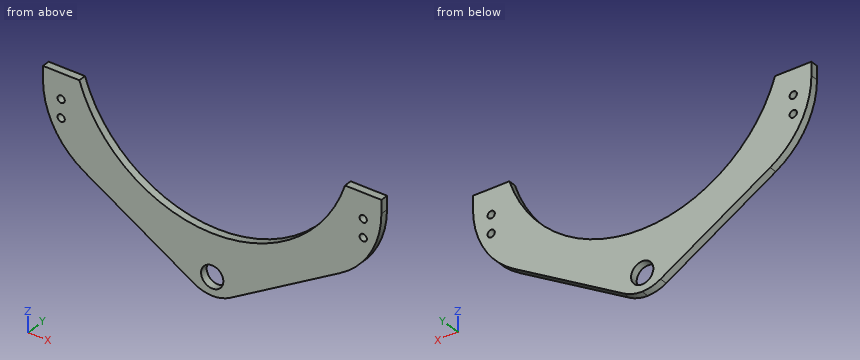
from build123d import *

# Parameters (mm, degrees)
SKETCH1_R           = 4.6
SKETCH1_R_2         = 1.5
BOSS_EXTRUDE2_DEPTH = 3.175


with BuildPart() as part:
    # Sketch1 → Boss-Extrude2 (new body)
    with BuildSketch(Plane(origin=(0, 0, 0), x_dir=(1, 0, 0), z_dir=(0, 1, 0))):
        with BuildLine():
            Line((109.700000056, 0), (117.200000056, 0))
            Line((117.200000056, 0), (124.700000056, 0))
            Line((124.700000056, 0), (124.700000056, 5.554920326))
            ThreePointArc((124.700000056, 5.554920326), (120.146392707, 22.818094267), (107.670447225, 35.589284453))
            Line((107.670447225, 35.589284453), (62.40678526, 62.67187034))
            ThreePointArc((62.40678526, 62.67187034), (58.77003956, 64.238725538), (54.850000028, 64.799300745))
            ThreePointArc((54.850000028, 64.799300745), (50.929960496, 64.238725538), (47.293214796, 62.67187034))
            Line((47.293214796, 62.67187034), (2.029552831, 35.589284453))
            ThreePointArc((2.029552831, 35.589284453), (-10.446392651, 22.818094267), (-15, 5.554920326))
            Line((-15, 5.554920326), (-15, 0))
            Line((-15, 0), (-7.5, 0))
            Line((-7.5, 0), (0, 0))
            ThreePointArc((0, 0), (54.850000028, 39.949878845), (109.700000056, 0))
        make_face()
        with Locations(Location((54.850000028, 57.3, 0), (0, 0, 270))):
            Circle(SKETCH1_R, mode=Mode.SUBTRACT)
        with BuildLine():
            ThreePointArc((117.200000056, 8.9), (115.700000056, 10.4), (117.200000056, 11.9))
            ThreePointArc((117.200000056, 11.9), (118.700000056, 10.4), (117.200000056, 8.9))
        make_face(mode=Mode.SUBTRACT)
        with Locations(Location((117.200000056, 17.9, 0), (0, 0, 270))):
            Circle(SKETCH1_R_2, mode=Mode.SUBTRACT)
        with BuildLine():
            ThreePointArc((-7.5, 8.9), (-9, 10.4), (-7.5, 11.9))
            ThreePointArc((-7.5, 11.9), (-6, 10.4), (-7.5, 8.9))
        make_face(mode=Mode.SUBTRACT)
        with Locations(Location((-7.5, 17.9, 0), (0, 0, 270))):
            Circle(SKETCH1_R_2, mode=Mode.SUBTRACT)
    extrude(amount=BOSS_EXTRUDE2_DEPTH)


solid = part.part
Verification items for the finished model (mm, model axes). Give positions to 0.01 mm unless a question says otherwise; leave off trailing zeros. Write each loop counter-clockwise with the first axis right and the second up, starting at its lowest first coordinate (ties: lowest second). Pieces come first, ordered by that corner, then holes.
(1) Cross-section at A-A (z = -23.5). Enter the section's corners in (x, y) (3 decimals).
(2) Material ranges on line 1 (X direction, y = 1.4, z = -10.4); line 2 (X direction, y = 0.7, z = -17.9); line 3 (X direction, y = 0.85, z = -12), recorded low to high.
(3) Gauge pin test, flat end, axial feed: pin 1 (12 mm diameter, centred on x = 54.85, z = -57.3, fed in from +Y) (3 decimals). Record the tip position at first contact, or that the pin passes through.
(4) Cross-section at C-C (z = -10.4). Enter the section's corners in (x, y) (3 decimals).
(5) Cross-section at D-D (z = -54). Enter the section's corners in (x, y) (3 decimals).
(6) Cross-section at B-B (y = 1.25). Enter the section's corners in (x, z).
Worked out:
1. outline: (-10.05, 0) - (14.534, 0) - (14.534, 3.175) - (-10.05, 3.175) - close; (95.166, 0) - (119.75, 0) - (119.75, 3.175) - (95.166, 3.175) - close
2. line 1: x = -14.66 to -9, -6 to 4.52, 105.18 to 115.7, 118.7 to 124.36
2. line 2: x = -12.75 to -9, -6 to 9.52, 100.18 to 115.7, 118.7 to 122.45
2. line 3: x = -14.4 to 5.45, 104.25 to 124.1
3. pin 1: stops at y = 3.175
4. outline: (-14.663, 0) - (-9, 0) - (-9, 3.175) - (-14.663, 3.175) - close; (-6, 0) - (4.525, 0) - (4.525, 3.175) - (-6, 3.175) - close; (105.175, 0) - (115.7, 0) - (115.7, 3.175) - (105.175, 3.175) - close; (118.7, 0) - (124.363, 0) - (124.363, 3.175) - (118.7, 3.175) - close
5. outline: (32.8, 0) - (51.645, 0) - (51.645, 3.175) - (32.8, 3.175) - close; (58.055, 0) - (76.9, 0) - (76.9, 3.175) - (58.055, 3.175) - close
6. outline: (-15, -5.55) arc R35 ccw to (2.03, -35.59) - (47.29, -62.67) arc R15 ccw to (54.85, -64.8) arc R15 ccw to (62.41, -62.67) - (107.67, -35.59) arc R35 ccw to (124.7, -5.55) - (124.7, 0) - (109.7, 0) arc R57.63 cw to (0, 0) - (-15, 0) - close; hole circle Ø3 at (-7.5, -17.9); hole circle Ø3 at (-7.5, -10.4); hole circle Ø9.2 at (54.85, -57.3); hole circle Ø3 at (117.2, -17.9); hole circle Ø3 at (117.2, -10.4)
